For this review, use the dimensioned drawing (mm, ordinates from the lowest corner) and the shaded views. Coordinates: 2 decimals unless noted, no trailing zeros. Write each loop counter-clockwise with the first axis right and the second up, starting at its lowest first coordinate (ties: lowest second). Pieces come first, ordered by that corner, then holes. Notation, with made-up numbers: (-13, 71) -> (34, 71) arc R13 cw to (34, 80) -> close; hole circle Ø1 at (-30, 77.25). An arc over 180 degrees is marked (long way). Put each result on its own line as item: value. Start each with the question number.
Item 1: Consider section D-D on x = 84.5. Give the boundary of the cut face in (y, z).
Item 2: Consider section B-B on y = 3. Give the boundary of the cut face in (x, z), and give its area (3 significant figures).
Item 3: Insertion check: P1, Ø1.5, axis at x = 89.5, z = 19.5, coming from the -Y side; P2, Ø2.5, axis at x = 75.5, y = 2, coming from the +Z side. Each pin has a flat end and moves straight along its axis. Give the tip position at first contact, or say it passes through.
Item 4: To check wall thickness, follow L1, parallel to X at y = 5.5, z = 7.5; L2, parallel to Z at x = 140, y = 5.25; L3, parallel to Z at x = 94, y = 4. State the ranges of each line that lie inside material, in increasing order.
Item 5: Consider section C-C on x = 20. Give the boundary of the cut face in (y, z).
Item 6: Consider section A-A on z = 7.5. Give the boundary of the cut face in (x, y).
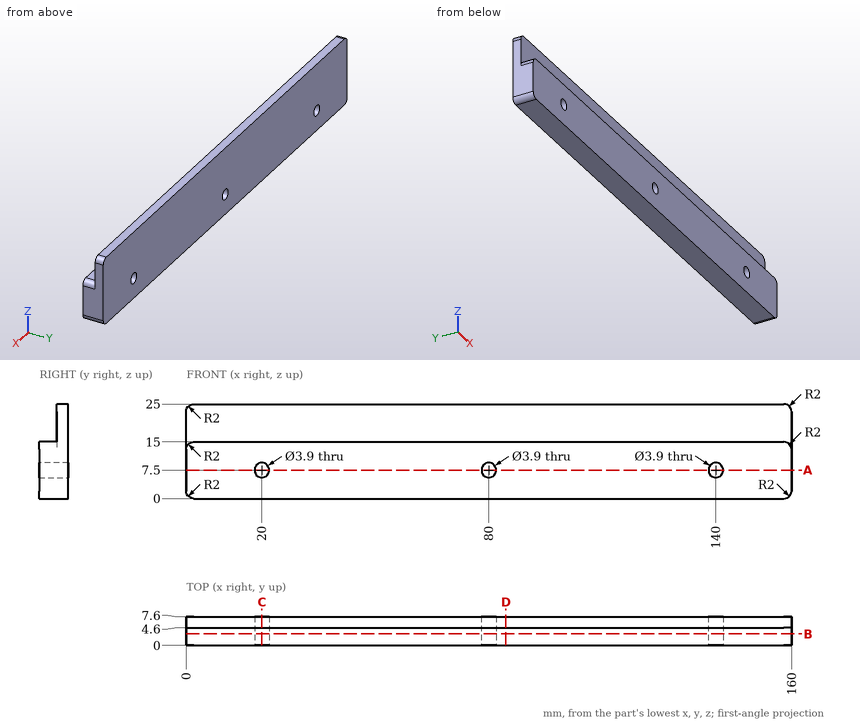
Return value:
1. outline: (0, 0) -> (7.6, 0) -> (7.6, 25) -> (4.6, 25) -> (4.6, 15) -> (0, 15) -> close
2. outline: (0, 2) arc R2 ccw to (2, 0) -> (158, 0) arc R2 ccw to (160, 2) -> (160, 13) arc R2 ccw to (158, 15) -> (2, 15) arc R2 ccw to (0, 13) -> close; hole circle Ø3.9 at (20, 7.5); hole circle Ø3.9 at (80, 7.5); hole circle Ø3.9 at (140, 7.5)
2. area: 2,360 mm^2
3. P1: y = 4.6
3. P2: z = 15
4. L1: 0 to 18.05, 21.95 to 78.05, 81.95 to 138.05, 141.95 to 160
4. L2: 0 to 5.55, 9.45 to 25
4. L3: 0 to 15
5. outline: (0, 0) -> (7.6, 0) -> (7.6, 5.55) -> (0, 5.55) -> close; (0, 9.45) -> (7.6, 9.45) -> (7.6, 25) -> (4.6, 25) -> (4.6, 15) -> (0, 15) -> close
6. outline: (0, 0) -> (18.05, 0) -> (18.05, 7.6) -> (0, 7.6) -> close; (21.95, 0) -> (78.05, 0) -> (78.05, 7.6) -> (21.95, 7.6) -> close; (81.95, 0) -> (138.05, 0) -> (138.05, 7.6) -> (81.95, 7.6) -> close; (141.95, 0) -> (160, 0) -> (160, 7.6) -> (141.95, 7.6) -> close
